Verification items for the finished model (mm, model axes). A direction names the side the tool comes from. Coordinates: 2 decimals unless noted, no trailing zeros. Write each loop counter-clockwise with the first axis right and the second up, starting at its lowest first coordinate (ties: lowest second). Pieces come first, ordered by that corner, then holes. Notation, with made-up numbers: M 1.5,14 L 24.5,14 A20 cw 24.5,37 Z; hole C -13,48.25 d10. An arc over 180 degrees is marked long. One line per item, written item: value.
```python
from build123d import *

# Parameters (mm, degrees)
ESBO_O1_W                                    = 150
ESBO_O1_H                                    = 31.75
RESSALTO_EXTRUS_O1_DEPTH                     = 12.7
ESBO_O2_W                                    = 150
ESBO_O2_H                                    = 9.525
RESSALTO_EXTRUS_O2_DEPTH                     = 75
ESBO_O4_R                                    = 4
CORTE_EXTRUS_O1_DEPTH                        = 117.483070122
REBAIXO_PARA_PARAFUSO_COM_CABE_A_PAN_2_COUNT = 2
REBAIXO_PARA_PARAFUSO_COM_CABE_A_PAN_2_PITCH = 70
ESBO_O7_R                                    = 3
CORTE_EXTRUS_O2_DEPTH                        = 9.525


# Read off the part's stored shape, not the designer's step: Rebaixo para parafuso com cabeça panela de M81
with BuildPart() as part:
    # Esboço1 → Ressalto-extrusão1 (new body)
    with BuildSketch(Plane.XY):
        Rectangle(ESBO_O1_W, ESBO_O1_H)
    extrude(amount=RESSALTO_EXTRUS_O1_DEPTH)

    # Esboço2 → Ressalto-extrusão2 (add)
    with BuildSketch(Plane.XY.offset(12.7)):
        with Locations((0, -11.1125)):
            Rectangle(ESBO_O2_W, ESBO_O2_H)
    extrude(amount=RESSALTO_EXTRUS_O2_DEPTH)

    # Esboço4 → Corte-extrusão1 (cut, through all)
    with BuildSketch(Plane(origin=(0, 0, 0), x_dir=(-1, 0, 0), z_dir=(0, 0, -1))):
        with Locations((-35, 0)):
            Circle(ESBO_O4_R)
        with Locations((35, 0)):
            Circle(ESBO_O4_R)
    extrude(amount=-CORTE_EXTRUS_O1_DEPTH, mode=Mode.SUBTRACT)

    # Esboço6 → Rebaixo para parafuso com cabe_a panela (revolve, cut)
    with BuildSketch(Plane(origin=(-35, 0, 12.7), x_dir=(0, -1, 0), z_dir=(1, 0, 0))):
        Polygon((0, 0), (0, 12.7), (3.3, 12.7), (3.3, 4.6), (6.5, 4.6), (6.5, 0.025), (6.525, 0), align=None)
    rebaixo_para_parafuso_com_cabe_a_panela = revolve(axis=Axis((-35, 0, 19.05), (0, 0, -1)), mode=Mode.SUBTRACT)

    # Rebaixo para parafuso com cabe_a pan 2: Rebaixo para parafuso com cabe_a panela ×2
    with Locations(*[(i * REBAIXO_PARA_PARAFUSO_COM_CABE_A_PAN_2_PITCH, 0, 0) for i in range(1, REBAIXO_PARA_PARAFUSO_COM_CABE_A_PAN_2_COUNT)]):
        add(rebaixo_para_parafuso_com_cabe_a_panela, mode=Mode.SUBTRACT)

    # Esboço7 → Corte-extrusão2 (cut)
    with BuildSketch(Plane.XZ.offset(15.875)):
        with Locations((-45, 62.7)):
            Circle(ESBO_O7_R)
        with Locations((45, 62.7)):
            Circle(ESBO_O7_R)
    extrude(amount=-CORTE_EXTRUS_O2_DEPTH, mode=Mode.SUBTRACT)

    # Rebaixo para parafuso com cabe_a pan 3 o → Rebaixo para parafuso com cabe_a pan 3 (revolve, cut)
    with BuildSketch(Plane(origin=(45, 0, 62.7), x_dir=(1, 0, 0), z_dir=(0, 0, 1))):
        Polygon((4.2, -9.875), (4.2, -6.35), (3, -6.35), (3, -15.875), (9.025, -15.875), (9, -15.85), (9, -9.875), align=None)
    revolve(axis=Axis((45, 0, 62.7), (0, 1, 0)), mode=Mode.SUBTRACT)

    # Rebaixo para parafuso com cabe_a pan 4 → Rebaixo para parafuso com cabe_a pan 3 2 (revolve, cut)
    with BuildSketch(Plane(origin=(-45, 0, 62.7), x_dir=(1, 0, 0), z_dir=(0, 0, 1))):
        Polygon((3, -15.875), (9.025, -15.875), (9, -15.85), (9, -9.875), (4.2, -9.875), (4.2, -6.35), (3, -6.35), align=None)
    revolve(axis=Axis((-45, 0, 62.7), (0, 1, 0)), mode=Mode.SUBTRACT)


solid = part.part
```
Item 1: Cross-section at A-A, the plane x = 45. Enter the section's corners in (y, z) (3 decimals).
The answers:
outline: M -15.875,0 L 15.875,0 L 15.875,12.7 L -6.35,12.7 L -6.35,58.5 L -9.875,58.5 L -9.875,53.7 L -15.85,53.7 L -15.875,53.675 Z; M -15.875,71.725 L -15.85,71.7 L -9.875,71.7 L -9.875,66.9 L -6.35,66.9 L -6.35,87.7 L -15.875,87.7 Z
Item 2: Scan lines: line 1 (Y direction, x = 35, z = 9.4) (3 decimals); line 2 (X direction, y = -8, z = 62); line 3 (Z direction, x = -45, y = -7.95). Record each from-to range of solid material in increasing order.
The answers:
line 1: y = -15.875 to -6.5, 6.5 to 15.875
line 2: x = -75 to -49.14, -40.86 to 40.86, 49.14 to 75
line 3: z = 0 to 58.5, 66.9 to 87.7
Item 3: Draft check along X on faces 1 (the face through (-1, 0, 0)), 2 (the face through (75, -7, 33)), 3 (the face through (32, 3, 8.1)), 4 (the face through (-75, -7, 33)). Enter one of: released by +X, released by -X, zero draft, split by the parting line, or undercut.
The answers:
face 1: zero draft
face 2: released by +X
face 3: undercut
face 4: released by -X
Item 4: Go/stop test with flat-tipped pins: P1, Ø13.5, axis at x = 45, z = 62.7, coming from the +Y side; P2, Ø14.5, axis at x = -45, z = 63, coming from the -Y side (3 decimals); P3, Ø10, axis at x = 59.5, y = 8, coming from the +Z side. Record where each tip stops, or that it passes through.
The answers:
P1: stops at y = -6.35
P2: stops at y = -9.875
P3: stops at z = 12.7
Item 5: Cross-section at B-B, the plane z = 62.7. Enter the section's corners in (x, y) (3 decimals), and give its area (3 significant figures).
The answers:
outline: M -75,-15.875 L -54.025,-15.875 L -54,-15.85 L -54,-9.875 L -49.2,-9.875 L -49.2,-6.35 L -75,-6.35 Z; M -40.8,-9.875 L -36,-9.875 L -36,-15.85 L -35.975,-15.875 L 35.975,-15.875 L 36,-15.85 L 36,-9.875 L 40.8,-9.875 L 40.8,-6.35 L -40.8,-6.35 Z; M 49.2,-9.875 L 54,-9.875 L 54,-15.85 L 54.025,-15.875 L 75,-15.875 L 75,-6.35 L 49.2,-6.35 Z
area: 1,150 mm²
Item 6: Access from +Z, -Z, +X, -X, +Y, -Y to the whole of each face (thin tool, end or side, straight path). Record for faces 5 (the face through (38.2, -2.4, 4)), 6 (the face through (-1, 5, 12.7)), 7 (the face through (43.049, -12.821, 71.486)).
The answers:
face 5: +Z, -Z
face 6: +Z, +X, -X, +Y
face 7: -Y
Item 7: Cross-section at D-D, the plane z = 14.5. Enter the section's corners in (x, y) (3 decimals), and give its area (3 significant figures).
The answers:
outline: M -75,-15.875 L 75,-15.875 L 75,-6.35 L -75,-6.35 Z
area: 1,430 mm²
Item 8: Cross-section at C-C, the plane x = -25.5. Enter the section's corners in (y, z) (3 decimals), and give its area (3 significant figures).
The answers:
outline: M -15.875,0 L 15.875,0 L 15.875,12.7 L -6.35,12.7 L -6.35,87.7 L -15.875,87.7 Z
area: 1,120 mm²
